Part model, mm, in its own coordinate system. A direction names the side the tool comes from. Give positions to 0.01 mm unless a question says otherwise; leave off trailing zeros. Write each loop counter-clockwise with the first axis right and the second up, starting at its lowest first coordinate (ties: lowest second). Pieces come first, ordered by that corner, then holes. Notation, with made-up numbers: M 62.25,-23.5 L 90.25,-23.5 A25 cw 90.25,2.5 Z; hole C 36,-9 d3. An arc over 180 degrees is marked long. Use a Markdown table: item, result.
```python
from build123d import *

# Parameters (mm, degrees)
F1_DEPTH = 63.5
F2_R     = 5.6131699843
F3_DEPTH = 107.696


# Not quite as in the source:
# - the program builds the solid bodies; features that only make, move or delete a surface that nothing else refers to are left out


with BuildPart() as f1:
    # F0 (on Front) → F1 (new body)
    with BuildSketch(Plane.XZ):
        Polygon((46.8248670694, 121.5258430131), (-35.8149119383, 25.0910623293), (31.6894345404, -32.7567829762), (48.2173903419, -13.4698268394), (0, 27.8500626645), (58.4593796701, 96.0680265203), (106.676770012, 54.7481370164), (386.0897425486, 54.7481370164), (420.2281583997, 94.5852552302), (488.444735815, 36.1270636701), (447.1248463111, -12.0903266718), (466.4118024479, -28.6182824733), (524.2596477533, 38.8860640054), (427.8248670694, 121.5258430131), align=None)
    extrude(amount=F1_DEPTH)

    # F2 (on face) → F3 (join)
    with BuildSketch(Plane(origin=(195.5607291239, 0, -167.5857540484), x_dir=(0, 1, 0), z_dir=(0.7593289818, 0, -0.6507069213))):
        with Locations((-31.75, 311.8531148615)):
            Circle(F2_R)
    extrude(amount=F3_DEPTH)


solid = f1.part
```
1. Drop flat-ended pins along their axis: P1, Ø6, axis at y = -51, z = -4.5, coming from the -X side (3 decimals); P2, Ø6, axis at y = -33.5, z = 81.5, coming from the +X side; P3, Ø12, axis at x = 417.5, z = 86, coming from the +Y side; P4, Ø5, axis at x = 259, y = -17, coming from the -Z side. Give the stop position or say it passes through.
Findings below:
| item | result |
|---|---|
| P1 | x = -4.785 |
| P2 | x = 478.03 |
| P3 | y = 0 |
| P4 | z = 54.75 |
2. Cut at C-C, the plane x = 454.5. State how many separate pieces and enclosed holes the cut face has, then the cut area to 3 significant figures.
Findings below:
| item | result |
|---|---|
| separate pieces | 3 |
| enclosed holes | 0 |
| area | 3,200 mm2 |
3. Drill centre lines: L1, parallel to X at y = -38, z = 80.5; L2, parallel to X at y = -48.5, z = 89; L3, parallel to X at y = -40.5, z = -22.5. Where is each one in solid material? Low to high.
Findings below:
| item | result |
|---|---|
| L1 | 11.67 to 45.12, 76.63 to 408.16, 436.66 to 475.7 |
| L2 | 18.95 to 52.4, 66.71 to 415.44, 426.75 to 465.78 |
| L3 | 19.72 to 40.48, 459.27 to 471.65 |
4. Cut at A-A, the plane z = 87. Give the cut face in (x, y), then the cut area to 3 significant figures.
Findings below:
| item | result |
|---|---|
| outline | M 17.24,-63.5 L 50.69,-63.5 L 50.69,0 L 17.24,0 Z; M 69.04,-63.5 L 413.73,-63.5 L 413.73,0 L 69.04,0 Z; M 429.08,-63.5 L 468.11,-63.5 L 468.11,0 L 429.08,0 Z |
| area | 26,500 mm2 |
5. Cut at D-D, the plane z = 109. Give the cut face in (x, y), then the cut area to 3 significant figures.
Findings below:
| item | result |
|---|---|
| outline | M 36.09,-63.5 L 442.44,-63.5 L 442.44,0 L 36.09,0 Z |
| area | 25,800 mm2 |
6. Tool access for faces 1 (the flat face through (453.859, -31.306, 65.765)), 2 (the flat face through (456.633, -31.306, -20.239)), 3 (the flat face through (494.93, -31.31, 4.66)): list every direction of +Z, -Z, +X, -X, +Y, -Y with a clear straight run to the whole face (end or side of a thin tool).
Findings below:
| item | result |
|---|---|
| face 1 | +Y, -Y |
| face 2 | -Z, +Y, -Y |
| face 3 | -Z, +X, +Y, -Y |
7. Cut at B-B, the plane y = -19.5. Give the cut face in (x, z), then the cut area to 3 significant figures.
Findings below:
| item | result |
|---|---|
| outline | M -35.81,25.09 L 31.69,-32.76 L 48.22,-13.47 L 0,27.85 L 58.46,96.07 L 106.68,54.75 L 386.09,54.75 L 420.23,94.59 L 488.44,36.13 L 447.12,-12.09 L 466.41,-28.62 L 524.26,38.89 L 427.82,121.53 L 46.82,121.53 Z |
| area | 32,100 mm2 |
